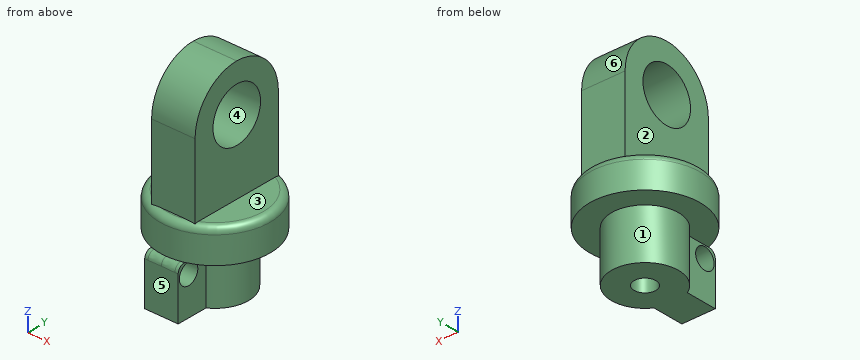
Solid Edge part; units mm, degrees
sketch "Sketch1" plane through (0, 0, 0) normal (0, 0, 1) x (1, 0, 0)
  circle A0 centre (0, 0) radius 9.75
extrude "Protrusion1" add sketch "Sketch1" along normal blind 31
sketch "Sketch2" plane through (0, 0, 0) normal (0, 0, -1) x (1, 0, 0)
  line L0 (-2.5, 4.3301) -> (-2.5, 9)
  line L1 (-2.5, 9) -> (2.5, 9)
  line L2 (2.5, 4.3301) -> (2.5, 9)
  arc A0 (2.5, 4.3301) -> (-2.5, 4.3301) centre (0, 0) cw
extrude "Extrusionsausschnitt_1" cut sketch "Sketch2" against normal blind 8 flip side to cut
sketch "Sketch3" plane through (0, 0, 31) normal (0, 0, 1) x (0, -1, 0)
  circle A0 centre (0, 0) radius 8.25
extrude "Extrusionsausschnitt_2" cut sketch "Sketch3" against normal blind 23 flip side to cut
hole "Bohrung_1" at (2.5, -7.25, 6.25) direction (-1, 0, 0) diameter 3.1 end up to next
sketch "Sketch4" plane through (0, 0, 31) normal (0, 0, 1) x (0, 1, 0)
  line L0 (-7, -3.25) -> (7, -3.25)
  line L1 (7, -3.25) -> (7, 3.25)
  line L2 (7, 3.25) -> (-7, 3.25)
  line L3 (-7, 3.25) -> (-7, -3.25)
  dimension "D1" = 7
  dimension "D2" = 7
extrude "Extrusionsausschnitt_3" cut sketch "Sketch4" against normal blind 18 flip side to cut
fillet "Verrundung_3" radius 7 2 edges at (0, -7, 31) (0, 7, 31)
sketch "Sketch5" plane through (3.25, 0, 22) normal (1, 0, 0) x (0, 1, 0)
  circle A0 centre (0, 2) radius 4
extrude "Extrusionsausschnitt_5" cut sketch "Sketch5" against normal blind 30
fillet "Verrundung_4" radius 1 1 edges at (-8.25, 0, 13)
sketch "Sketch6" plane through (0, 0, 0) normal (1, 0, 0) x (0, 1, 0)
  line L0 (-9.424, 0.5) -> (5, 0.5)
extrude "Extrusionsausschnitt_6" cut sketch "Sketch6" along normal mid plane 852 material side at (0, -2.212, 0.45)
fillet "Verrundung_5" radius 1 1 edges at (0, -9, 8)
hole "Bohrung_2" at (0, 0, 0.5) direction (0, 0, 1) diameter 3.242 depth 12
The listing builds one solid part. Answer for the finished solid, in the listing's coordinates (mm). Face numbers are marked on the shaded views. A direction names the side the tool comes from. Coordinates: 2 decimals unless noted, no trailing zeros. Write each loop counter-clockwise with the first axis right and the second up, starting at its lowest first coordinate (ties: lowest second). Pieces come first, ordered by that corner, then holes. Notation, with made-up numbers: M -5,46 L 16,46 A21 cw 16,51 Z; hole C -7,11 d9. An arc over 180 degrees is marked long. Put each result on its own line as item: value. Start each with the question number.
1. Flat-ended cylindrical pins translate along their axes: P1, Ø1.5, axis at y = 0, z = 17.5, coming from the -X side; P2, Ø1.2, axis at x = -6, y = -2.5, coming from the +Z side; P3, Ø1, axis at x = 5, z = 10.5, coming from the +Y side. Find the tip coordinate at first contact, or state that the pin passes through.
2. A cutting plane is placed at C-C on x = 1.25. Count the separate pieces of the cut face and the enclosed holes in it, then the cut area to 3 significant figures.
3. For a pull along Z with two mould halves and no side action, classify the marked faces 4, 5 and 6 as pulls with the +Z half, pulls with the -Z half, needs draft (parallel to the pull), parting line crosses it, or undercut.
4. Consider line 1 (Z direction, x = -0.5, y = 0); line 2 (Z direction, x = -1.3, y = -7.25); line 3 (Y direction, x = 0.5, z = 5). Determine where each line is inside the solid, lowest interval first. Write a range as from..to.
5. A cutting plane is placed at B-B on z = 22. Write down the section's boundary in (x, y), then the cut area to 3 significant figures.
6. A cutting plane is placed at D-D on z = 10. Write down the section's boundary in (x, y).
7. A cutting plane is placed at A-A on z = 6.25. Write down the section's boundary in (x, y), then the cut area to 3 significant figures.
8. Which of the six approach directions +Z, -Z, +X, -X, +Y, -Y give full straight-line access (tool end or side, diameter ignored) to the marked faces 1, 2 and 3?
Resolved:
1. P1: stops at x = -3.25
1. P2: stops at z = 13
1. P3: stops at y = 6.91
2. separate pieces: 1
2. enclosed holes: 2
2. area: 333 mm2
3. face 4: undercut
3. face 5: needs draft
3. face 6: pulls with the +Z half
4. line 1: z = 12.5..20, 28..31
4. line 2: z = 0.5..4.7, 7.8..12.99
4. line 3: y = -9..-8.17, -6.33..-1.54, 1.54..4.97
5. outline: M -3.25,-7 L 3.25,-7 L 3.25,-3.46 L -3.25,-3.46 Z; M -3.25,3.46 L 3.25,3.46 L 3.25,7 L -3.25,7 Z
5. area: 46.0 mm2
6. outline: C 0,0 d16.5; hole C 0,0 d3.24
7. outline: M -2.5,-9 L 2.5,-9 L 2.5,-8.8 L -2.5,-8.8 Z; M -2.5,-5.7 L 2.5,-5.7 L 2.5,-4.33 A5 ccw long -2.5,-4.33 Z; hole C 0,0 d3.24
7. area: 75.9 mm2
8. face 1: -Z
8. face 2: +Z, -X, +Y, -Y
8. face 3: +Z, +X, +Y, -Y
